Part model, mm, in its own coordinate system. A direction names the side the tool comes from. Coordinates: 2 decimals unless noted, no trailing zeros. Write each loop counter-clockwise with the first axis right and the second up, starting at its lowest first coordinate (ties: lowest second). Pieces come first, ordered by that corner, then holes. Notation, with made-up numbers: M 73.5,71.25 L 90.5,71.25 A28 cw 90.5,96.25 Z; hole C 2,78 d6. An arc over 180 degrees is marked long. Use a Markdown table: item, result. Add a question column.
Q1. Slice it at A-A on x = 25.5. Write the cut outline in (y, z) (3 decimals), then the cut area to 3 significant figures.
Q2. Wall check: L1, parallel to Y at x = -281, z = 9 (3 decimals); L2, parallel to Y at x = -514.35, z = -0.95; L3, parallel to Z at x = 156.5, y = -17 (3 decimals). Give the ranges that are in metal, low to high. Write a range as from..to.
Q3. Pin check, flat tips, straight feed: pin 1 Ø1.9 at (y, z) = (-34.5, 12) entering from +X; pin 2 Ø1.6 at (x, z) = (-561.5, -1) entering from +Y; pin 3 Ø9 at (x, y) = (336.55, -19.05) entering from +Z. Stop position of each tip, or through.
Q4. Mould opens along Y. For faces 3 (the flat face through (-8, 0, -3.175)), 4 (the flat face through (8, 0, 0)), 5 (the flat face through (8, 38.1, 20)), 6 (the flat face through (-8, -34.925, 21)) say: released by +Y, released by -Y, zero draft, split by the parting line, or undercut.
Q5. Tool access for faces 1 (the flat face through (-8, -38.1, 20)), 2 (the flat face through (8, 34.925, 21)): list every direction of +Z, -Z, +X, -X, +Y, -Y with a clear straight run to the whole face (end or side of a thin tool).
from build123d import *

# Parameters (mm, degrees)
SKETCH1_W                        = 1079.5
SKETCH1_H                        = 63.5
BASE_FLANGE1_DEPTH               = 3.175
EDGE_FLANGE4_DEPTH               = 1079.5
EDGE_FLANGE4_BEND_DEPTH          = 1079.5
EDGE_FLANGE1_DEPTH               = 63.5
EDGE_FLANGE1_BEND_DEPTH          = 63.5
F_17_64_0_26563_DIAMETER_HOLE1_D = 6.747002
F_11_32_0_34375_DIAMETER_HOLE1_D = 8.73125
CUT_EXTRUDE1_DEPTH               = 600.469933045
FILLET1_R                        = 3.175
F_17_64_0_26563_DIAMETER_HOLE2_D = 6.747002
F_17_64_0_26563_DIAMETER_HOLE3_D = 6.747002


# Sheet-metal steps are written as plain solids
with BuildPart() as part:
    # Sketch1 → Base-Flange1 (new body)
    with BuildSketch(Plane.XY):
        Rectangle(SKETCH1_W, SKETCH1_H)
    extrude(amount=-BASE_FLANGE1_DEPTH)

    # Edge-Flange4 section (across the edge) → Edge-Flange4 (add)
    with BuildSketch(Plane(origin=(-539.75, -34.925, 0), x_dir=(0, 1, 0), z_dir=(1, 0, 0))):
        with BuildLine():
            Line((-3.175, 3.175), (-3.175, 38.1))
            Line((-3.175, 38.1), (0, 38.1))
            Line((0, 38.1), (0, 3.175))
            ThreePointArc((0, 3.175), (0.92993597, 0.92993597), (3.175, 0))
            Line((3.175, 0), (3.175, -3.175))
            ThreePointArc((3.175, -3.175), (-1.315128061, -1.315128061), (-3.175, 3.175))
        make_face()
    extrude(amount=EDGE_FLANGE4_DEPTH)

    # Edge-Flange4 section 2 (across the edge) → Edge-Flange4 bend (add)
    with BuildSketch(Plane(origin=(539.75, 34.925, 0), x_dir=(0, -1, 0), z_dir=(-1, 0, 0))):
        with BuildLine():
            Line((-3.175, 3.175), (-3.175, 38.1))
            Line((-3.175, 38.1), (0, 38.1))
            Line((0, 38.1), (0, 3.175))
            ThreePointArc((0, 3.175), (0.92993597, 0.92993597), (3.175, 0))
            Line((3.175, 0), (3.175, -3.175))
            ThreePointArc((3.175, -3.175), (-1.315128061, -1.315128061), (-3.175, 3.175))
        make_face()
    extrude(amount=EDGE_FLANGE4_BEND_DEPTH)

    # Edge-Flange1 section (across the edge) → Edge-Flange1 (add)
    with BuildSketch(Plane(origin=(-590.55, 31.75, 0), x_dir=(1, 0, 0), z_dir=(0, -1, 0))):
        with BuildLine():
            Line((-3.175, 3.175), (-3.175, 44.45))
            Line((-3.175, 44.45), (0, 44.45))
            Line((0, 44.45), (0, 3.175))
            ThreePointArc((0, 3.175), (0.92993597, 0.92993597), (3.175, 0))
            Line((3.175, 0), (50.8, 0))
            Line((50.8, 0), (50.8, -3.175))
            Line((50.8, -3.175), (3.175, -3.175))
            ThreePointArc((3.175, -3.175), (-1.315128061, -1.315128061), (-3.175, 3.175))
        make_face()
    extrude(amount=EDGE_FLANGE1_DEPTH)

    # Edge-Flange1 section 2 (across the edge) → Edge-Flange1 bend (add)
    with BuildSketch(Plane(origin=(590.55, -31.75, 0), x_dir=(-1, 0, 0), z_dir=(0, 1, 0))):
        with BuildLine():
            Line((-3.175, 3.175), (-3.175, 44.45))
            Line((-3.175, 44.45), (0, 44.45))
            Line((0, 44.45), (0, 3.175))
            ThreePointArc((0, 3.175), (0.92993597, 0.92993597), (3.175, 0))
            Line((3.175, 0), (50.8, 0))
            Line((50.8, 0), (50.8, -3.175))
            Line((50.8, -3.175), (3.175, -3.175))
            ThreePointArc((3.175, -3.175), (-1.315128061, -1.315128061), (-3.175, 3.175))
        make_face()
    extrude(amount=EDGE_FLANGE1_BEND_DEPTH)

    # 17/64 (0.26563) Diameter Hole1 (through all)
    with Locations(Plane(origin=(0, 0, -3.175), x_dir=(-1, 0, 0), z_dir=(0, 0, -1))):
        with Locations((-565.15, 0), (565.15, 0)):
            Hole(F_17_64_0_26563_DIAMETER_HOLE1_D / 2)

    # 11/32 (0.34375) Diameter Hole1 (through all)
    with Locations(Plane(origin=(0, 0, -3.175), x_dir=(-1, 0, 0), z_dir=(0, 0, -1))):
        with Locations((-276.225, 0), (276.225, 0)):
            Hole(F_11_32_0_34375_DIAMETER_HOLE1_D / 2)

    # Sketch50 → Cut-Extrude1 (cut, through all)
    with BuildSketch(Plane(origin=(0, 31.75, 0), x_dir=(1, 0, 0), z_dir=(0, 1, 0))):
        with BuildLine():
            Line((590.55, -3.175), (590.55, -44.45))
            Line((590.55, -44.45), (593.725, -44.45))
            Line((593.725, -44.45), (593.725, -3.175))
            ThreePointArc((593.725, -3.175), (591.865128061, 1.315128061), (587.375, 3.175))
            Line((587.375, 3.175), (587.375, 0))
            ThreePointArc((587.375, 0), (589.62006403, -0.92993597), (590.55, -3.175))
        make_face()
        with BuildLine():
            Line((-593.725, -3.175), (-593.725, -44.45))
            Line((-593.725, -44.45), (-590.55, -44.45))
            Line((-590.55, -44.45), (-590.55, -3.175))
            ThreePointArc((-590.55, -3.175), (-589.62006403, -0.92993597), (-587.375, 0))
            Line((-587.375, 0), (-587.375, 3.175))
            ThreePointArc((-587.375, 3.175), (-591.865128061, 1.315128061), (-593.725, -3.175))
        make_face()
    extrude(amount=-CUT_EXTRUDE1_DEPTH, mode=Mode.SUBTRACT)

    # Fillet1
    fillet1_edges = [part.edges().sort_by_distance(p)[0] for p in [
        (-539.75, -36.5125, 38.1),
        (539.75, -36.5125, 38.1),
        (539.75, 36.5125, 38.1),
        (-539.75, 36.5125, 38.1),
        (-587.375, 31.75, -1.5875),
        (-587.375, -31.75, -1.5875),
        (587.375, -31.75, -1.5875),
        (587.375, 31.75, -1.5875),
    ]]
    fillet(fillet1_edges, radius=FILLET1_R)

    # 17/64 (0.26563) Diameter Hole2 (through all)
    with Locations(Plane(origin=(0, 38.1, 0), x_dir=(1, 0, 0), z_dir=(0, 1, 0))):
        with Locations((-528.6375, -7.9375), (-528.6375, -30.1625), (-176.2125, -30.1625), (-176.2125, -7.9375), (176.2125, -7.9375), (176.2125, -30.1625), (528.6375, -7.9375), (528.6375, -30.1625)):
            Hole(F_17_64_0_26563_DIAMETER_HOLE2_D / 2)

    # 17/64 (0.26563) Diameter Hole3 (through all)
    with Locations(Plane(origin=(0, 0, -3.175), x_dir=(-1, 0, 0), z_dir=(0, 0, -1))):
        with Locations((-514.35, 19.05), (-514.35, -19.05), (-336.55, 19.05), (-336.55, -19.05), (336.55, 19.05), (336.55, -19.05), (514.35, 19.05), (514.35, -19.05)):
            Hole(F_17_64_0_26563_DIAMETER_HOLE3_D / 2)


solid = part.part
Recorded:
| question | item | result |
|---|---|---|
| 1 | outline | M -38.1,3.175 A6.35 ccw -31.75,-3.175 L 31.75,-3.175 A6.35 ccw 38.1,3.175 L 38.1,38.1 L 34.925,38.1 L 34.925,3.175 A3.175 cw 31.75,0 L -31.75,0 A3.175 cw -34.925,3.175 L -34.925,38.1 L -38.1,38.1 Z |
| 1 | area | 471 mm² |
| 2 | L1 | -38.1..-34.925, 34.925..38.1 |
| 2 | L2 | -36.58..-22.42, -15.68..15.68, 22.42..36.58 |
| 2 | L3 | -3.175..0 |
| 3 | pin 1 | x = 539.75 |
| 3 | pin 2 | y = 31.75 |
| 3 | pin 3 | z = 0 |
| 4 | face 3 | zero draft |
| 4 | face 4 | undercut |
| 4 | face 5 | released by +Y |
| 4 | face 6 | undercut |
| 5 | face 1 | +Z, -Z, +X, -X, -Y |
| 5 | face 2 | +Z, +X, -X |
